Can you work these out from the model? Positions are in its coordinate system, mm. Face numbers are marked on the shaded views. Round coordinates to 2 decimals unless told otherwise and drop trailing zeros. Write each loop counter-clockwise with the first axis right and the second up, starting at its lowest first coordinate (ties: lowest second). Pieces come first, ordered by that corner, then holes. Notation, with made-up numbers: (-12, -37) - (23, -37) arc R17 cw to (23, -22) - close; hole circle Ø3 at (34, 52.25). An arc over 180 degrees is marked (long way). One line per item, written item: value. Start each with the question number.
(1) I want a section at C-C on z = 22.5. List the corners of the cut face in (x, y) for me.
(2) If I drill on L1, parallel to X at y = 24, z = 11; L2, parallel to Y at x = 25.5, z = 14.5; L3, parallel to Y at x = -26, z = 17.5, over which ranges is the centre line in solid material (lowest first)? Write a range as from..to.
(3) Thinking about a two-plate mould opening in X: for the marked faces 1, 2 and 3, which applies, +X half, -X half, draft (parallel to the pull), parting line (faces both ways), or undercut?
(4) I want a section at A-A on y = 0. List the corners of the cut face in (x, z) for me, plus the area to 3 significant figures.
(5) I'm going to push flat-ended pins straight in: pin 1 Ø4 at (y, z) = (-9, 17.5) entering from +X; pin 2 Ø1.5 at (x, z) = (3, 15.5) entering from +Y; pin 3 Ø3 at (x, y) = (26, -24) entering from -Z (1 decimal); pin 4 Ø6 at (x, z) = (-14, 27) entering from +Y. Where does each tip first touch, or does it pass through?
from build123d import *

# Parameters (mm, degrees)
SKETCH001_R = 1.75
PAD_DEPTH   = 40


with BuildPart() as part:
    # Sketch → Revolution (revolve)
    with BuildSketch(Plane.XZ):
        Polygon((38, 0), (38, 40), (39, 40), (39, 39), (40, 39), (40, 0), align=None)
    revolve(axis=Axis((0, 0, 0), (0, 0, 1)))

    # Sketch001 → Pad (new body)
    with BuildSketch(Plane(origin=(0, 0, 0), x_dir=(1, 0, 0), z_dir=(0, 0, -1))):
        with BuildLine():
            ThreePointArc((23.9651596918, 26.2044103339), (23.7955896661, 21.9651596918), (28.0348403082, 21.7955896661))
            Line((28.0348403082, 21.7955896661), (29.957371204, 23.57023357))
            Line((29.957371204, 23.57023357), (25.8876905876, 27.9790542377))
            Line((25.8876905876, 27.9790542377), (23.9651596918, 26.2044103339))
        make_face()
        with Locations((26, 24)):
            Circle(SKETCH001_R, mode=Mode.SUBTRACT)
        with BuildLine():
            ThreePointArc((28.0348403082, -21.7955896661), (23.7955896661, -21.9651596918), (23.9651596918, -26.2044103339))
            Line((25.8876905876, -27.9790542377), (23.9651596918, -26.2044103339))
            Line((29.957371204, -23.57023357), (25.8876905876, -27.9790542377))
            Line((28.0348403082, -21.7955896661), (29.957371204, -23.57023357))
        make_face()
        with Locations((26, -24)):
            Circle(SKETCH001_R, mode=Mode.SUBTRACT)
    pad = extrude(amount=-PAD_DEPTH)

    # Mirrored: Pad across Sketch001 V_Axis
    add(pad.mirror(Plane(origin=(0, 0, 0), x_dir=(0, 0, -1), z_dir=(1, 0, 0))))


solid = part.part
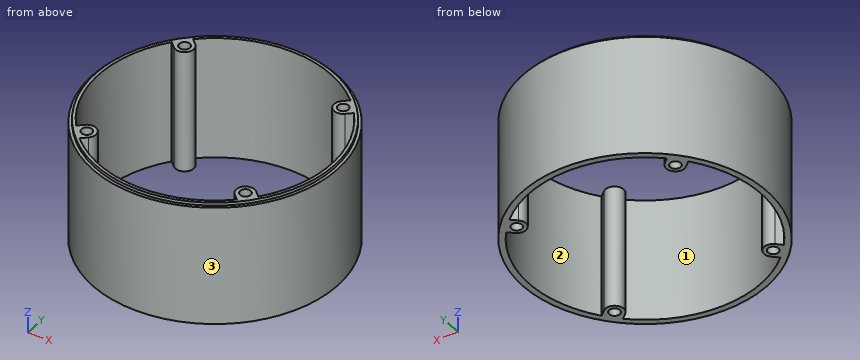
Established:
1. outline: circle Ø80 at (0, 0); hole (-29.87, -23.49) - (-28.03, -21.8) arc R3 cw to (-23.97, -26.2) - (-25.8, -27.9) arc R38 ccw to (25.8, -27.9) - (23.97, -26.2) arc R3 cw to (28.03, -21.8) - (29.87, -23.49) arc R38 ccw to (29.87, 23.49) - (28.03, 21.8) arc R3 cw to (23.97, 26.2) - (25.8, 27.9) arc R38 ccw to (-25.8, 27.9) - (-23.97, 26.2) arc R3 cw to (-28.03, 21.8) - (-29.87, 23.49) arc R38 ccw to start; hole circle Ø3.5 at (-26, -24); hole circle Ø3.5 at (-26, 24); hole circle Ø3.5 at (26, -24); hole circle Ø3.5 at (26, 24)
2. L1: -32..-27.75, -24.25..-23, 23..24.25, 27.75..32
2. L2: -30.82..-28.17, -27.62..-25.68, -22.32..-21.04, 21.04..22.32, 25.68..27.62, 28.17..30.82
2. L3: -30.4..-25.75, -22.25..-21, 21..22.25, 25.75..30.4
3. face 1: undercut
3. face 2: undercut
3. face 3: parting line
4. outline: (-40, 0) - (-38, 0) - (-38, 40) - (-39, 40) - (-39, 39) - (-40, 39) - close; (38, 0) - (40, 0) - (40, 39) - (39, 39) - (39, 40) - (38, 40) - close
4. area: 158 mm2
5. pin 1: x = 39.38
5. pin 2: y = 39.94
5. pin 3: through
5. pin 4: y = 38.46
